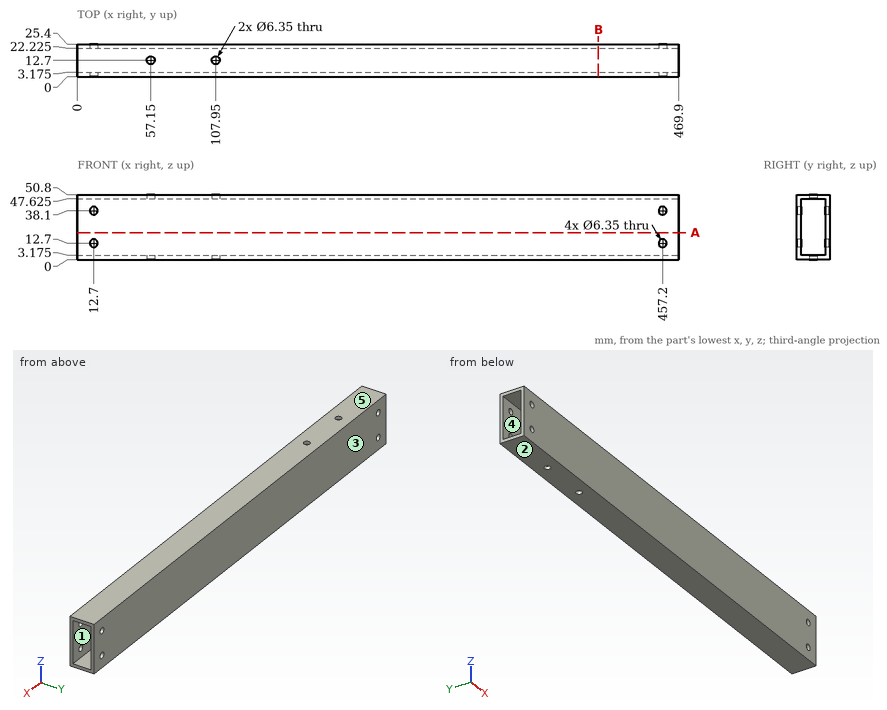
Print and shaded views of the part. All mm, measured from the part's lowest x, y and z. A direction names the side the tool comes from. Coordinates: 2 decimals unless noted, no trailing zeros. Order: outer loops, then holes, each group sorted by start corner. A loop starts at its lowest first (then second) coordinate and runs counter-clockwise, first axis right, second up. Notation, with made-up numbers: (-18.75, -13.75) - (9.25, -13.75) arc R31 cw to (9.25, 21.25) - close; hole circle Ø11 at (-23, 25). An arc over 180 degrees is marked (long way). Put each result on its own line as item: value.
1. Saw through at B-B (x = 407). Write the cut outline in (y, z) (3 decimals).
Answer sheet:
outline: (0, 0) - (25.4, 0) - (25.4, 50.8) - (0, 50.8) - close; hole (3.175, 3.175) - (22.225, 3.175) - (22.225, 47.625) - (3.175, 47.625) - close
2. Tool access for the marked faces 4 and 5: list every direction of +Z, -Z, +X, -X, +Y, -Y with a clear straight run to the whole face (end or side of a thin tool).
Answer sheet:
face 4: +X, -X
face 5: +Z, +X, -X, +Y, -Y
3. Drop a flat-ended pin along its axis: P1, Ø5, axis at x = 457.2, z = 12.7, coming from the +Y side. Give the stop position or say it passes through.
Answer sheet:
P1: passes through
4. Saw through at A-A (z = 21). Write the cut outline in (x, y) (3 decimals), and give its area (3 significant figures).
Answer sheet:
outline: (0, 0) - (469.9, 0) - (469.9, 3.175) - (0, 3.175) - close; (0, 22.225) - (469.9, 22.225) - (469.9, 25.4) - (0, 25.4) - close
area: 2,980 mm^2
5. Pull direction Z, two halves, no side cores. Call the marked faces 1, 2 and 3: pulls with the +Z half, pulls with the -Z half, needs draft (parallel to the pull), parting line crosses it, or undercut.
Answer sheet:
face 1: undercut
face 2: pulls with the -Z half
face 3: needs draft
6. Probe line 1 along X through (y, z) = (23.8, 38.1) (3 decimals); line 2 along Z through (x, y) = (457.2, 2.2) (3 decimals); line 3 along Y through (x, z) = (57.15, 49) (3 decimals). List the from-to ranges inside material, lowest first. Write a range as [from, to].
Answer sheet:
line 1: x = [0, 9.525], [15.875, 454.025], [460.375, 469.9]
line 2: z = [0, 9.525], [15.875, 34.925], [41.275, 50.8]
line 3: y = [0, 9.525], [15.875, 25.4]
